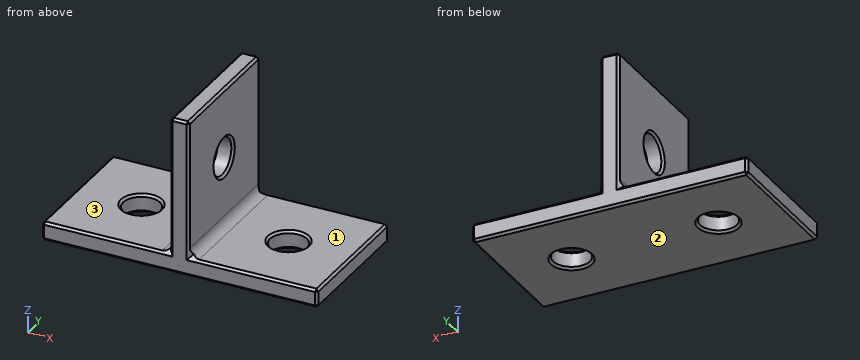
from build123d import *

# Parameters (mm, degrees)
SKETCH_W           = 30
SKETCH_H           = 15
PAD_DEPTH          = 2
SKETCH001_W        = 2
SKETCH001_H        = 15
PAD001_DEPTH       = 15
SKETCH002_R        = 2
POCKET_DEPTH       = 2
POLARPATTERN_COUNT = 2
SKETCH003_R        = 2
POCKET001_DEPTH    = 2
CHAMFER_SIZE       = 0.25
FILLET_R           = 1


with BuildPart() as part:
    # Sketch → Pad (new body)
    with BuildSketch(Plane.XY):
        Rectangle(SKETCH_W, SKETCH_H)
    extrude(amount=PAD_DEPTH)

    # Sketch001 (on Face6 of Pad) → Pad001 (join)
    with BuildSketch(Plane.XY.offset(2)):
        Rectangle(SKETCH001_W, SKETCH001_H)
    extrude(amount=PAD001_DEPTH)

    # Sketch002 (on Face5 of Pad001) → Pocket (cut)
    with BuildSketch(Plane.XY.offset(2)):
        with Locations((8, 0)):
            Circle(SKETCH002_R)
    pocket = extrude(amount=-POCKET_DEPTH, mode=Mode.SUBTRACT)

    # PolarPattern: Pocket ×2 about axis
    polarpattern_axis = Axis((0, 0, 2), (0, 0, 1))
    for i in range(1, POLARPATTERN_COUNT):
        add(pocket.rotate(polarpattern_axis, i * 360 / POLARPATTERN_COUNT), mode=Mode.SUBTRACT)

    # Sketch003 (on Face9 of PolarPattern) → Pocket001 (cut)
    with BuildSketch(Plane.YZ.offset(1)):
        with Locations((0, 9.5)):
            Circle(SKETCH003_R)
    extrude(amount=-POCKET001_DEPTH, mode=Mode.SUBTRACT)

    # Chamfer
    chamfer_edges = [part.edges().sort_by_distance(p)[0] for p in [
        (-6, 0, 2),
        (6, 0, 2),
        (-1, -2, 9.5),
        (1, -2, 9.5),
        (-1, 0, 17),
        (1, 0, 17),
        (0, -7.5, 17),
        (0, 7.5, 17),
        (-1, 7.5, 9.5),
        (1, 7.5, 9.5),
        (8, 7.5, 2),
        (-8, 7.5, 2),
        (0, 7.5, 0),
        (-15, 0, 2),
        (15, 0, 2),
        (6, 0, 0),
        (-6, 0, 0),
        (-8, -7.5, 2),
        (-1, -7.5, 9.5),
        (1, -7.5, 9.5),
        (0, -7.5, 0),
        (15, -7.5, 1),
        (8, -7.5, 2),
        (-15, -7.5, 1),
        (-15, 7.5, 1),
        (-15, 0, 0),
        (15, 7.5, 1),
        (15, 0, 0),
    ]]
    chamfer(chamfer_edges, length=CHAMFER_SIZE)

    # Fillet
    fillet_edges = [part.edges().sort_by_distance(p)[0] for p in [
        (1, 0, 2),
        (-1, 0, 2),
    ]]
    fillet(fillet_edges, radius=FILLET_R)


solid = part.part
Design review of the part built by this model. Coordinates are the model's own, in mm. Face numbers are marked on the shaded views. A direction names the side the tool comes from. Coordinates: 2 decimals unless noted, no trailing zeros. Write each loop counter-clockwise with the first axis right and the second up, starting at its lowest first coordinate (ties: lowest second). Pieces come first, ordered by that corner, then holes. Notation, with made-up numbers: (40, 35) -> (75, 35) arc R5 ccw to (75, 42) -> close; hole circle Ø5 at (34.25, 48.25). An arc over 180 degrees is marked (long way). Write each question's results on one line, items separated by ' | '. Start each with the question number.
(1) Take a section at B-B on z = 9.5. Write out the cut boundary in (x, y).
(2) Take a section at D-D on y = -3.5. Write out the cut boundary in (x, z).
(3) Tool access review of the marked faces 1, 2 and 3: name each direction out of +Z, -Z, +X, -X, +Y, -Y from which nothing blocks a thin tool from reaching the whole face with its end or side.
(4) Take a section at C-C on z = 1. Write out the cut boundary in (x, y), and give its area (3 significant figures).
(5) Clearance check with flat-ended pins moving along their axes: P1, Ø3, axis at x = -6, y = -1, coming from the +Z side; P2, Ø2, axis at y = 2.5, z = 9.5, coming from the -X side; P3, Ø3, axis at y = 0, z = 9.5, coming from the -X side. State where each tip first meets the part, or that it passes through.
(6) Take a section at A-A on x = -8. Write out the cut boundary in (y, z).
(7) For line 1 along Y through (x, z) = (-8, 1.25); line 2 along Z through (x, y) = (0.2, 0); line 3 along Z through (x, y) = (5.5, -5), list the stretches that pass through material, from the lowest coordinate up. Write a range as from..to.
Results found:
1) outline: (-1, -7.25) -> (-0.75, -7.5) -> (0.75, -7.5) -> (1, -7.25) -> (1, -2.25) -> (0.75, -2) -> (-0.75, -2) -> (-1, -2.25) -> close; (-1, 2.25) -> (-0.75, 2) -> (0.75, 2) -> (1, 2.25) -> (1, 7.25) -> (0.75, 7.5) -> (-0.75, 7.5) -> (-1, 7.25) -> close
2) outline: (-15, 0.25) -> (-14.75, 0) -> (14.75, 0) -> (15, 0.25) -> (15, 1.75) -> (14.75, 2) -> (2, 2) arc R1 cw to (1, 3) -> (1, 16.75) -> (0.75, 17) -> (-0.75, 17) -> (-1, 16.75) -> (-1, 3) arc R1 cw to (-2, 2) -> (-14.75, 2) -> (-15, 1.75) -> close
3) face 1: +Z, +X, +Y, -Y | face 2: -Z, +X, -X, +Y, -Y | face 3: +Z, -X, +Y, -Y
4) outline: (-15, -7.25) -> (-14.75, -7.5) -> (14.75, -7.5) -> (15, -7.25) -> (15, 7.25) -> (14.75, 7.5) -> (-14.75, 7.5) -> (-15, 7.25) -> close; hole circle Ø4 at (-8, 0); hole circle Ø4 at (8, 0) | area: 425 mm2
5) P1: stops at z = 2 | P2: stops at x = -1 | P3: passes through
6) outline: (-7.5, 0.25) -> (-7.25, 0) -> (-2.25, 0) -> (-2, 0.25) -> (-2, 1.75) -> (-2.25, 2) -> (-7.25, 2) -> (-7.5, 1.75) -> close; (2, 0.25) -> (2.25, 0) -> (7.25, 0) -> (7.5, 0.25) -> (7.5, 1.75) -> (7.25, 2) -> (2.25, 2) -> (2, 1.75) -> close
7) line 1: y = -7.5..-2, 2..7.5 | line 2: z = 0..7.5, 11.5..17 | line 3: z = 0..2
